For this review, take the finished solid that the model builds, in its own axes (mm). Face numbers are marked on the shaded views. Coordinates: 2 decimals unless noted, no trailing zeros. Write each loop counter-clockwise with the first axis right and the second up, starting at its lowest first coordinate (ties: lowest second). Pieces come first, ordered by that corner, then holes.
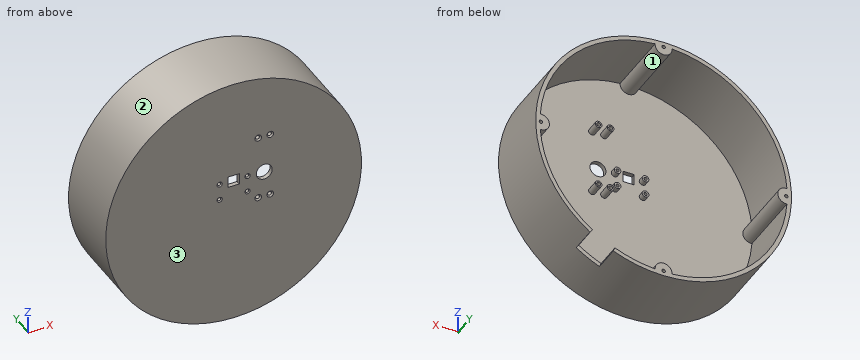
```python
from build123d import *

# Parameters (mm, degrees)
SKETCH1_R                                            = 96
BOSS_EXTRUDE1_DEPTH                                  = 53.975
SKETCH2_R                                            = 1.3208
CUT_EXTRUDE1_DEPTH                                   = 50.8
SKETCH3_R                                            = 6
SKETCH3_W                                            = 8.5
SKETCH3_H                                            = 8.5
CUT_EXTRUDE2_DEPTH                                   = 145.957373045
BOSS_EXTRUDE2_START                                  = 3.175
BOSS_EXTRUDE2_OUTLINE_R                              = 2.5
BOSS_EXTRUDE2_DEPTH                                  = 4.325
BOSS_EXTRUDE3_START                                  = 3.175
BOSS_EXTRUDE3_OUTLINE_R                              = 2.5
BOSS_EXTRUDE3_DEPTH                                  = 9.652
CSK_FOR_M2_5_CROSS_COUNTERSUNK_HEAD_SCRE_D           = 2.9
CSK_FOR_M2_5_CROSS_COUNTERSUNK_HEAD_SCRE_CSINK_D     = 5
CSK_FOR_M2_5_CROSS_COUNTERSUNK_HEAD_SCRE_CSINK_ANGLE = 92
CSK_FOR_M2_CROSS_COUNTERSUNK_HEAD_SCREW1_D           = 2.4
CSK_FOR_M2_CROSS_COUNTERSUNK_HEAD_SCREW1_CSINK_D     = 4
CSK_FOR_M2_CROSS_COUNTERSUNK_HEAD_SCREW1_CSINK_ANGLE = 92
CUT_EXTRUDE4_DEPTH                                   = 20


# Read off the part's stored shape, not the designer's step: Boss-Extrude2, Boss-Extrude3
with BuildPart() as part:
    # Sketch1 → Boss-Extrude1 (new body)
    with BuildSketch(Plane(origin=(0, 0, 0), x_dir=(1, 0, 0), z_dir=(0, 1, 0))):
        with Locations(Location((0, 0, 0), (0, 0, 270))):
            Circle(SKETCH1_R)
    extrude(amount=BOSS_EXTRUDE1_DEPTH)

    # Sketch2 → Cut-Extrude1 (cut)
    with BuildSketch(Plane(origin=(0, 53.975, 0), x_dir=(1, 0, 0), z_dir=(0, 1, 0))):
        with Locations(Location((0, 92.075, 0), (0, 0, 270))):
            Circle(SKETCH2_R)
        with Locations(Location((92.075, 0, 0), (0, 0, 270))):
            Circle(SKETCH2_R)
        with Locations(Location((0, -92.075, 0), (0, 0, 270))):
            Circle(SKETCH2_R)
        with Locations(Location((-92.075, 0, 0), (0, 0, 270))):
            Circle(SKETCH2_R)
        with BuildLine():
            Line((92.609089058, 6.327499417), (92.607548963, 6.35))
            ThreePointArc((92.607548963, 6.35), (65.629212709, 65.64516025), (6.327499417, 92.609089058))
            ThreePointArc((6.327499417, 92.609089058), (0, 85.725), (-6.327499417, 92.609089058))
            ThreePointArc((-6.327499417, 92.609089058), (-65.637186964, 65.637186964), (-92.609089058, 6.327499417))
            ThreePointArc((-92.609089058, 6.327499417), (-85.725, 0), (-92.609089058, -6.327499417))
            Line((-92.609089058, -6.327499417), (-92.607548963, -6.35))
            ThreePointArc((-92.607548963, -6.35), (-65.629212709, -65.64516025), (-6.327499417, -92.609089058))
            ThreePointArc((-6.327499417, -92.609089058), (0, -85.725), (6.327499417, -92.609089058))
            Line((6.327499417, -92.609089058), (6.35, -92.607548963))
            ThreePointArc((6.35, -92.607548963), (65.64516025, -65.629212709), (92.609089058, -6.327499417))
            ThreePointArc((92.609089058, -6.327499417), (85.725, 0), (92.609089058, 6.327499417))
        make_face()
    extrude(amount=-CUT_EXTRUDE1_DEPTH, mode=Mode.SUBTRACT)

    # Sketch3 → Cut-Extrude2 (cut, through all)
    with BuildSketch(Plane(origin=(0, 3.175, 0), x_dir=(1, 0, 0), z_dir=(0, 1, 0))):
        with Locations(Location((23, -16.5546, 0), (0, 0, 270))):
            Circle(SKETCH3_R)
        with Locations((0, -16.8926)):
            Rectangle(SKETCH3_W, SKETCH3_H)
    extrude(amount=-CUT_EXTRUDE2_DEPTH, mode=Mode.SUBTRACT)

    # Boss-Extrude2 outline → Boss-Extrude2 (add)
    with BuildSketch(Plane(origin=(0, 0, 0), x_dir=(1, 0, 0), z_dir=(0, 1, 0)).offset(BOSS_EXTRUDE2_START)):
        with Locations((10.5, -4.4926)):
            Circle(BOSS_EXTRUDE2_OUTLINE_R)
        with Locations((10.5, -16.9926)):
            Circle(BOSS_EXTRUDE2_OUTLINE_R)
        with Locations((-10.5, -16.9926)):
            Circle(BOSS_EXTRUDE2_OUTLINE_R)
        with Locations((-10.5, -4.4926)):
            Circle(BOSS_EXTRUDE2_OUTLINE_R)
    extrude(amount=BOSS_EXTRUDE2_DEPTH)

    # Boss-Extrude3 outline → Boss-Extrude3 (add)
    with BuildSketch(Plane(origin=(0, 0, 0), x_dir=(1, 0, 0), z_dir=(0, 1, 0)).offset(BOSS_EXTRUDE3_START)):
        with Locations((27.5, 3.3254)):
            Circle(BOSS_EXTRUDE3_OUTLINE_R)
        with Locations((18.5, -45.6746)):
            Circle(BOSS_EXTRUDE3_OUTLINE_R)
        with Locations((27.5, -45.6746)):
            Circle(BOSS_EXTRUDE3_OUTLINE_R)
        with Locations((18.5, 3.3254)):
            Circle(BOSS_EXTRUDE3_OUTLINE_R)
    extrude(amount=BOSS_EXTRUDE3_DEPTH)

    # CSK for M2.5 Cross Countersunk Head Screw1 (through all)
    with Locations(Plane(origin=(0, 0, 0), x_dir=(-1, 0, 0), z_dir=(0, -1, 0))):
        with Locations((-27.5, 3.3254), (-18.5, 3.3254), (-27.5, -45.6746), (-18.5, -45.6746)):
            CounterSinkHole(CSK_FOR_M2_5_CROSS_COUNTERSUNK_HEAD_SCRE_D / 2, CSK_FOR_M2_5_CROSS_COUNTERSUNK_HEAD_SCRE_CSINK_D / 2, counter_sink_angle=CSK_FOR_M2_5_CROSS_COUNTERSUNK_HEAD_SCRE_CSINK_ANGLE)

    # CSK for M2 Cross Countersunk Head Screw1 (through all)
    with Locations(Plane(origin=(0, 0, 0), x_dir=(-1, 0, 0), z_dir=(0, -1, 0))):
        with Locations((10.5, -4.4926), (-10.5, -4.4926), (-10.5, -16.9926), (10.5, -16.9926)):
            CounterSinkHole(CSK_FOR_M2_CROSS_COUNTERSUNK_HEAD_SCREW1_D / 2, CSK_FOR_M2_CROSS_COUNTERSUNK_HEAD_SCREW1_CSINK_D / 2, counter_sink_angle=CSK_FOR_M2_CROSS_COUNTERSUNK_HEAD_SCREW1_CSINK_ANGLE)

    # Sketch10 → Cut-Extrude4 (cut)
    with BuildSketch(Plane(origin=(0, 53.975, 0), x_dir=(1, 0, 0), z_dir=(0, 1, 0))):
        with BuildLine():
            Line((37.80459918, 88.242916321), (36.554290822, 85.324465703))
            ThreePointArc((36.554290822, 85.324465703), (45.243395364, 81.052549626), (53.440238661, 75.898758335))
            Line((53.440238661, 75.898758335), (55.268116471, 78.494810667))
            ThreePointArc((55.268116471, 78.494810667), (46.790907136, 83.824882996), (37.80459918, 88.242916321))
        make_face()
    extrude(amount=-CUT_EXTRUDE4_DEPTH, mode=Mode.SUBTRACT)


solid = part.part
```
Q1. Draft analysis for pull direction Z (two halves, no side actions). For the marked faces 1, 2 and 3, state which applies: +Z half, -Z half, draft (parallel to the pull), parting line (faces both ways), or undercut.
Ans:
face 1: undercut
face 2: parting line
face 3: draft
Q2. Add section A-A (y = 51). Give the number of separate pieces and of enclosed holes in the cut face, then the cut area to 3 significant figures.
Ans:
separate pieces: 1
enclosed holes: 4
area: 2,090 mm2
Q3. Clearance check with flat-ended pins moving along their axes: pin 1 Ø10 at (x, y) = (-31.5, 31.5) entering from -Z; pin 2 Ø4.5 at (x, z) = (27.5, 45.67) entering from -Y; pin 3 Ø4 at (x, z) = (18.5, 45.67) entering from +Y; pin 4 Ø7 at (x, z) = (23, 16.55) entering from -Y. State where each tip first meets the part, or that it passes through.
Ans:
pin 1: stops at z = -92.27
pin 2: stops at y = 0.24
pin 3: stops at y = 12.83
pin 4: passes through
Q4. Add section C-C (z = 35). State the section outline as (x, y) points (3 decimals), then the cut area to 3 significant figures.
Ans:
outline: (-89.392, 0) - (89.392, 0) - (89.392, 53.975) - (85.974, 53.975) - (85.974, 3.175) - (-85.974, 3.175) - (-85.974, 53.975) - (-89.392, 53.975) - close
area: 915 mm2
Q5. For probe 1 along Z at (x, y) = (-10.5, 2.75); probe 2 along Z at (x, y) = (-10.5, 5.75); probe 3 along X at (y, z) = (4.5, 44), list the stretches that pass through material, from the lowest coordinate up.
Ans:
probe 1: z = -95.42 to 3.29, 5.69 to 15.79, 18.19 to 95.42
probe 2: z = -95.42 to -92.23, 1.99 to 3.29, 5.69 to 6.99, 14.49 to 15.79, 18.19 to 19.49, 92.23 to 95.42
probe 3: x = -85.32 to -81.73, 16.64 to 20.36, 25.64 to 29.36, 81.73 to 85.32
Q6. Add section B-B (x = 34). State the section outline as (y, z) points (1 decimal).
Ans:
outline: (0, -89.8) - (54, -89.8) - (54, -86.4) - (3.2, -86.4) - (3.2, 86.4) - (54, 86.4) - (54, 89.8) - (0, 89.8) - close
